```python
from build123d import *

# Parameters (mm, degrees)
SKETCH1_R               = 1.5
BASE_EXTRUDE_DEPTH      = 12
BASE_EXTRUDE_DEPTH_BACK = 0.0001
CUT_EXTRUDE1_DEPTH      = 1.799999969
CUT_EXTRUDE1_TAPER      = 2


with BuildPart() as part:
    # Sketch1 → Base-Extrude (new body, two sides)
    with BuildSketch(Plane.XY) as base_extrude_sk:
        Circle(SKETCH1_R)
    extrude(amount=BASE_EXTRUDE_DEPTH)
    extrude(base_extrude_sk.sketch, amount=-BASE_EXTRUDE_DEPTH_BACK)

    # Sketch6 → Boss-Revolve2 (revolve)
    with BuildSketch(Plane(origin=(0, 0, 0), x_dir=(1, 0, 0), z_dir=(0, 1, 0))):
        with BuildLine():
            Line((0, -12), (2.7999999, -12))
            Line((2.7999999, -12), (2.7999999, -13.54246308))
            ThreePointArc((2.7999999, -13.54246308), (1.46418655, -14.180811406), (0, -14.4))
            Line((0, -14.4), (0, -12))
        make_face()
    revolve(axis=Axis((0, 0, -0.393620135), (0, 0, 1)))

    # Sketch7 → Cut-Extrude1 (cut)
    with BuildSketch(Plane(origin=(0, 0, 14.7000001), x_dir=(-1, 0, 0), z_dir=(0, 0, -1))):
        with BuildLine():
            ThreePointArc((0.205000004, 1.48592565), (0, 1.500000013), (-0.205000004, 1.48592565))
            Line((-0.205000004, 1.48592565), (-0.205000004, 0.708178558))
            ThreePointArc((-0.205000004, 0.708178558), (-0.35072876, 0.355344481), (-0.702967546, 0.208182689))
            Line((-0.702967546, 0.208182689), (-1.48592565, 0.205000004))
            ThreePointArc((-1.48592565, 0.205000004), (-1.500000013, 0), (-1.48592565, -0.205000004))
            Line((-1.48592565, -0.205000004), (-0.702967546, -0.208182689))
            ThreePointArc((-0.702967546, -0.208182689), (-0.35072876, -0.355344481), (-0.205000004, -0.708178558))
            Line((-0.205000004, -0.708178558), (-0.205000004, -1.48592565))
            ThreePointArc((-0.205000004, -1.48592565), (0, -1.500000013), (0.205000004, -1.48592565))
            Line((0.205000004, -1.48592565), (0.205000004, -0.708178558))
            ThreePointArc((0.205000004, -0.708178558), (0.35072876, -0.355344481), (0.702967546, -0.208182689))
            Line((0.702967546, -0.208182689), (1.48592565, -0.205000004))
            ThreePointArc((1.48592565, -0.205000004), (1.500000013, 0), (1.48592565, 0.205000004))
            Line((1.48592565, 0.205000004), (0.702967546, 0.208182689))
            ThreePointArc((0.702967546, 0.208182689), (0.35072876, 0.355344481), (0.205000004, 0.708178558))
            Line((0.205000004, 0.708178558), (0.205000004, 1.48592565))
        make_face()
    extrude(amount=CUT_EXTRUDE1_DEPTH, taper=CUT_EXTRUDE1_TAPER, mode=Mode.SUBTRACT)


solid = part.part
```
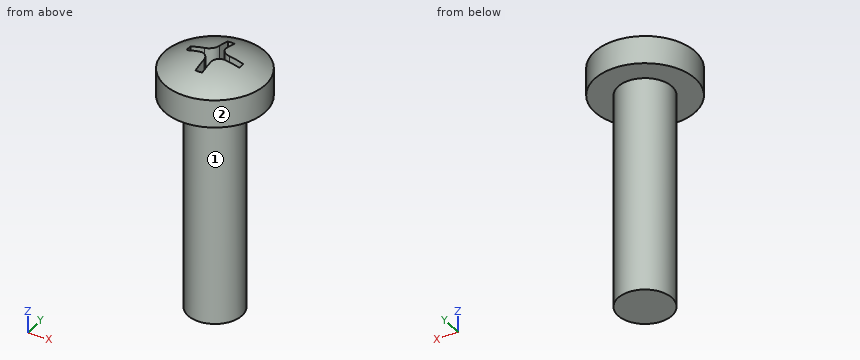
Geometry check sheet. Reference: the model listing, model coordinates, mm. Face numbers are marked on the shaded views. A direction names the side the tool comes from. Coordinates: 2 decimals unless noted, no trailing zeros. Order: outer loops, then holes, each group sorted by start corner. A loop starts at its lowest first (then second) coordinate and runs counter-clockwise, first axis right, second up. Notation, with made-up numbers: M 73.5,9 L 82.5,9 A27 ccw 82.5,27 Z; hole C 46.25,62.5 d9. An arc over 180 degrees is marked long. One line per question, with ' | ' between items. Start each with the question number.
Item 1: Material ranges on L1, parallel to X at y = -0.3, z = 4; L2, parallel to Z at x = 0.35, y = 0.2; L3, parallel to Z at x = 0.55, y = 0.6, recorded low to high. Write a range as [from, to].
Item 2: Cross-section at B-B on z = 9.5. Enter the section's corners in (x, y), then the cut area to 3 significant figures.
Item 3: Set-up check for the marked faces 1 and 2: record each of +Z, -Z, +X, -X, +Y, -Y from which the full face is reachable in a straight line by a thin tool's end or side.
Item 4: Gauge pin test, flat ends, axial feed: pin 1 (2 mm diameter, centred on x = -1.5, z = 8, fed in from -Y); pin 2 (2.5 mm diameter, centred on x = -0.5, y = 0.5, fed in from +Z); pin 3 (1 mm diameter, centred on y = -1, z = 4.5, fed in from -X). Record the tip position at first contact, or that the pin passes through.
Item 5: Cross-section at A-A on y = -2.2. Enter the section's corners in (x, z).
Findings:
1) L1: x = [-1.47, 1.47] | L2: z = [0, 12.9] | L3: z = [0, 14.33]
2) outline: C 0,0 d3 | area: 7.07 mm²
3) face 1: -Z | face 2: +Z, -Z
4) pin 1: stops at y = -1.41 | pin 2: stops at z = 14.38 | pin 3: stops at x = -1.41
5) outline: M -1.73,12 L 1.73,12 L 1.73,13.54 A4.49 ccw -1.73,13.54 Z
